Input: part model. Units: mm. Frame: model coordinates. Face numbers are marked on the shaded views. Round coordinates to 2 decimals unless told otherwise and drop trailing zeros. Order: outer loops, then holes, each group sorted by start corner. A loop starts at its lowest first (then second) coordinate and runs counter-clockwise, first axis right, second up. Notation, with made-up numbers: (57, -20.75) -> (65, -20.75) arc R27 cw to (65, 7.25) -> close; hole circle Ø10 at (44, -19.75). An arc over 180 degrees is marked (long way). Use a Markdown table: item, result.
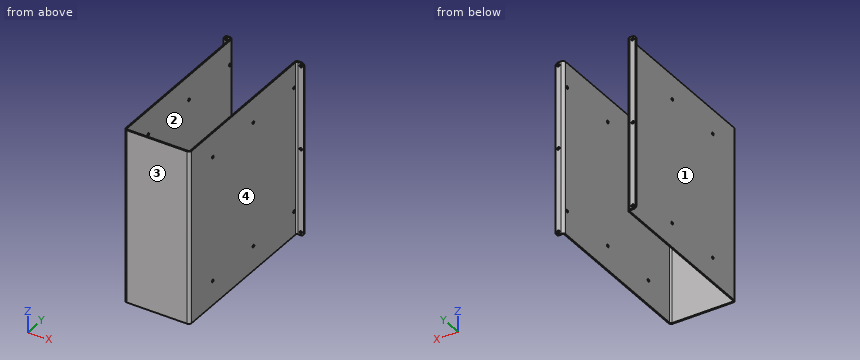
from build123d import *

# Parameters (mm, degrees)
F1_DEPTH = 234.95
F2_R     = 3.69316
F3_R     = 1.98374
F4_R     = 3.96875
F5_R     = 1.8288
F6_DEPTH = 89.11082
F7_R     = 1.8288
F8_DEPTH = 1.70942


with BuildPart() as f1:
    # F0 (on Top) → F1 (new body)
    with BuildSketch(Plane.XY):
        Polygon((0, -225.18116), (0, 0), (-11.63066, 0), (-11.63066, -1.70942), (-1.70942, -1.70942), (-1.70942, -226.89058), (87.4014, -226.89058), (87.4014, -1.70942), (97.32264, -1.70942), (97.32264, 0), (85.69198, 0), (85.69198, -225.18116), align=None)
    extrude(amount=F1_DEPTH)

    # F2
    f2_edges = [f1.edges().sort_by_distance(p)[0] for p in [
        (-1.70942, -226.89058, 117.475),
        (87.4014, -226.89058, 117.475),
        (85.69198, 0, 117.475),
        (0, 0, 117.475),
    ]]
    fillet(f2_edges, radius=F2_R)

    # F3
    f3_edges = [f1.edges().sort_by_distance(p)[0] for p in [
        (0, -225.18116, 117.475),
        (85.69198, -225.18116, 117.475),
        (-1.70942, -1.70942, 117.475),
        (87.4014, -1.70942, 117.475),
    ]]
    fillet(f3_edges, radius=F3_R)

    # F4
    f4_edges = [f1.edges().sort_by_distance(p)[0] for p in [
        (-11.63066, -0.85471, 0),
        (-11.63066, -0.85471, 234.95),
        (97.32264, -0.85471, 234.95),
        (97.32264, -0.85471, 0),
    ]]
    fillet(f4_edges, radius=F4_R)

    # F5 (on face) → F6 (cut, through all)
    with BuildSketch(Plane.YZ.offset(87.4014)):
        with Locations((-6.86816, 33.061364)):
            Circle(F5_R)
        with Locations((-92.600069, 33.061364)):
            Circle(F5_R)
        with Locations((-178.331978, 33.061364)):
            Circle(F5_R)
        with Locations((-178.331978, 201.888636)):
            Circle(F5_R)
        with Locations((-92.600069, 201.888636)):
            Circle(F5_R)
        with Locations((-6.86816, 201.888636)):
            Circle(F5_R)
    extrude(amount=-F6_DEPTH, mode=Mode.SUBTRACT)

    # F7 (on face) → F8 (cut, through all)
    with BuildSketch(Plane(origin=(0, 0, 0), x_dir=(-1, 0, 0), z_dir=(0, 1, 0))):
        with Locations((-93.35389, 3.96875)):
            Circle(F7_R)
        with Locations((-93.35389, 117.475)):
            Circle(F7_R)
        with Locations((-93.35389, 230.98125)):
            Circle(F7_R)
        with Locations((7.66191, 230.98125)):
            Circle(F7_R)
        with Locations((7.66191, 117.475)):
            Circle(F7_R)
        with Locations((7.66191, 3.96875)):
            Circle(F7_R)
    extrude(amount=-F8_DEPTH, mode=Mode.SUBTRACT)


solid = f1.part
1) Cut plane B-B on z = 163.5. Return loops of the section in (x, y).
Answer key:
| item | result |
|---|---|
| outline | (-11.63, -1.71) -> (-3.69, -1.71) arc R1.98 cw to (-1.71, -3.69) -> (-1.71, -223.2) arc R3.69 ccw to (1.98, -226.89) -> (83.71, -226.89) arc R3.69 ccw to (87.4, -223.2) -> (87.4, -3.69) arc R1.98 cw to (89.39, -1.71) -> (97.32, -1.71) -> (97.32, 0) -> (89.39, 0) arc R3.69 ccw to (85.69, -3.69) -> (85.69, -223.2) arc R1.98 cw to (83.71, -225.18) -> (1.98, -225.18) arc R1.98 cw to (0, -223.2) -> (0, -3.69) arc R3.69 ccw to (-3.69, 0) -> (-11.63, 0) -> close |
2) Cut plane A-A on y = -53. Return loops of the section in (x, z), and give its area (3 significant figures).
Answer key:
| item | result |
|---|---|
| outline | (-1.71, 0) -> (0, 0) -> (0, 234.95) -> (-1.71, 234.95) -> close; (85.69, 0) -> (87.4, 0) -> (87.4, 234.95) -> (85.69, 234.95) -> close |
| area | 803 mm^2 |
3) Cut plane C-C on x = 47. Return loops of the section in (y, z), and give its area (3 significant figures).
Answer key:
| item | result |
|---|---|
| outline | (-226.89, 0) -> (-225.18, 0) -> (-225.18, 234.95) -> (-226.89, 234.95) -> close |
| area | 402 mm^2 |
4) Contact query for flat-ended pins moving along their axis: P1, Ø4, axis at y = -92.6, z = 201.89, coming from the -X side; P2, Ø4, axis at x = 95, z = 119.5, coming from the -Y side; P3, Ø2, axis at y = -141.5, z = 149.5, coming from the +X side. Output: stop coordinate, or through.
Answer key:
| item | result |
|---|---|
| P1 | stops at x = -1.71 |
| P2 | stops at y = -1.71 |
| P3 | stops at x = 87.4 |
5) Ray query, probe 1 along X at (y, z) = (-174.5, 212); probe 2 along Y at (x, z) = (49, 205.5); probe 3 along Y at (x, z) = (-3.5, 43.5). Return the intervals inside material, ascending.
Answer key:
| item | result |
|---|---|
| probe 1 | x = -1.71 to 0, 85.69 to 87.4 |
| probe 2 | y = -226.89 to -225.18 |
| probe 3 | y = -1.72 to -0.01 |
6) Draft query along X for the marked faces 1, 2, 3 and 4. Return one class per face: released by +X, released by -X, zero draft, split by the parting line, or undercut.
Answer key:
| item | result |
|---|---|
| face 1 | released by -X |
| face 2 | undercut |
| face 3 | zero draft |
| face 4 | released by +X |
